```python
from build123d import *

# Parameters (mm, degrees)
BOSS_EXTRUDE1_DEPTH = 20
FILLET1_R           = 10


with BuildPart() as part:
    # Sketch1 → Boss-Extrude1 (new body)
    with BuildSketch(Plane(origin=(0, 0, 0), x_dir=(1, 0, 0), z_dir=(0, 1, 0))):
        with BuildLine():
            Line((-20, -150), (20, -150))
            ThreePointArc((20, -150), (41.213203436, -141.213203436), (50, -120))
            Line((50, -120), (50, 120))
            ThreePointArc((50, 120), (41.213203436, 141.213203436), (20, 150))
            Line((20, 150), (-20, 150))
            ThreePointArc((-20, 150), (-41.213203436, 141.213203436), (-50, 120))
            Line((-50, 120), (-50, -120))
            ThreePointArc((-50, -120), (-41.213203436, -141.213203436), (-20, -150))
        make_face()
    extrude(amount=BOSS_EXTRUDE1_DEPTH)

    # Fillet1
    fillet1_edges = [part.edges().sort_by_distance(p)[0] for p in [
        (-41.213203436, 20, 141.213203436),
        (0, 20, 150),
        (41.213203436, 20, 141.213203436),
        (50, 20, 0),
        (41.213203436, 20, -141.213203436),
        (0, 20, -150),
        (-41.213203436, 20, -141.213203436),
        (-50, 20, 0),
    ]]
    fillet(fillet1_edges, radius=FILLET1_R)


solid = part.part
```
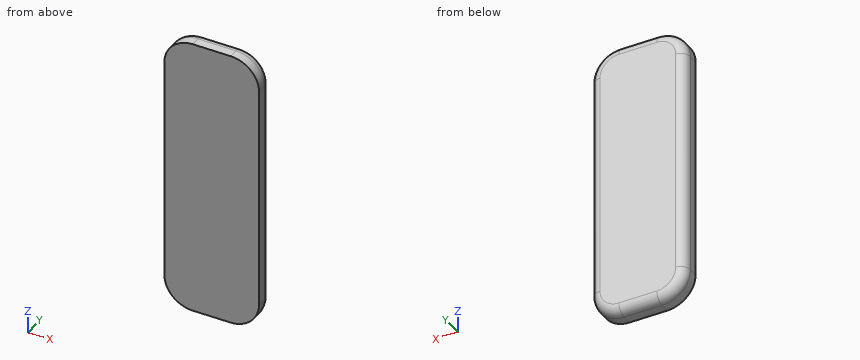
CAD build for the part. Positions are in the model's coordinates, mm. Coordinates: 2 decimals unless noted, no trailing zeros. Loops run counter-clockwise (first coordinate to the right, second up) from the corner with the lowest first, then second, coordinate; pieces in that order, holes last. Notation, with made-up numbers: (-4, -24) - (34, -24) arc R10 ccw to (34, -5) - close; hole circle Ø1 at (75.5, -31). An arc over 180 degrees is marked (long way). Use CSV: the item, a comma, the result in double quotes. Start each with the question number.
Q1. Drop flat-ended pins along their axis: P1, Ø4, axis at y = 13, z = 33, coming from the -X side; P2, Ø1, axis at x = -27.5, y = 16, coming from the -Z side; P3, Ø1.5, axis at x = -8, y = 14, coming from the -Z side. Give the stop position or say it passes through.
Q2. Cut at B-B, the plane y = 3.25. List the corners of the cut face in (x, z), then the cut area to 3 significant figures.
Q3. Cut at C-C, the plane y = 15.75. List the corners of the cut face in (x, z), then the cut area to 3 significant figures.
Q4. Cut at A-A, the plane z = -1. List the corners of the cut face in (x, y).
Q5. Probe probe 1 along Z at (x, y) = (-4.5, 10.5); probe 2 along Z at (x, y) = (1, 13.75); probe 3 along X at (y, z) = (15.75, 49). List the from-to ranges inside material, lowest first. Write a range as from..to.
Here are the results:
1,P1,"x = -49.95"
1,P2,"z = -147.37"
1,P3,"z = -149.46"
2,outline,"(-50, -120) arc R30 ccw to (-20, -150) - (20, -150) arc R30 ccw to (50, -120) - (50, 120) arc R30 ccw to (20, 150) - (-20, 150) arc R30 ccw to (-50, 120) - close"
2,area,"29,200 mm2"
3,outline,"(-48.18, -120) arc R28.18 ccw to (-20, -148.18) - (20, -148.18) arc R28.18 ccw to (48.18, -120) - (48.18, 120) arc R28.18 ccw to (20, 148.18) - (-20, 148.18) arc R28.18 ccw to (-48.18, 120) - close"
3,area,"27,900 mm2"
4,outline,"(-50, 0) - (50, 0) - (50, 10) arc R10 ccw to (40, 20) - (-40, 20) arc R10 ccw to (-50, 10) - close"
5,probe 1,"-149.99..149.99"
5,probe 2,"-149.27..149.27"
5,probe 3,"-48.18..48.18"
